CAD build for the part. Positions are in the model's coordinates, mm. A direction names the side the tool comes from. Give positions to 0.01 mm unless a question says otherwise; leave off trailing zeros. Write each loop counter-clockwise with the first axis right and the second up, starting at its lowest first coordinate (ties: lowest second). Pieces come first, ordered by that corner, then holes. Notation, with made-up numbers: (38, -15.5) - (76, -15.5) arc R8 cw to (76, -8.5) - close; hole circle Ø4 at (10.25, -20.75). An arc over 180 degrees is marked (long way). Answer as a JSON object with one key per item and string values.
from build123d import *

# Parameters (mm, degrees)
F0_W     = 461.772
F0_H     = 76.2
F1_DEPTH = 35.814
F2_W     = 62.3316
F2_H     = 31.496
F3_DEPTH = 461.773


with BuildPart() as f1:
    # F0 (on Top) → F1 (new body)
    with BuildSketch(Plane.XY):
        with Locations((-38.690397, 9.206371)):
            Rectangle(F0_W, F0_H)
    extrude(amount=F1_DEPTH)

    # F2 (on face) → F3 (cut, through all)
    with BuildSketch(Plane(origin=(-269.576397, 0, 0), x_dir=(0, -1, 0), z_dir=(-1, 0, 0))):
        with Locations((-9.206371, 20.066)):
            Rectangle(F2_W, F2_H)
    extrude(amount=-F3_DEPTH, mode=Mode.SUBTRACT)


solid = f1.part
(1) Saw through at B-B, the plane x = 6.5. Give the cut face in (y, z).
Answer key:
{"outline": "(-28.89, 0) - (47.31, 0) - (47.31, 35.81) - (40.37, 35.81) - (40.37, 4.32) - (-21.96, 4.32) - (-21.96, 35.81) - (-28.89, 35.81) - close"}
(2) Pull direction Y, two halves, no side cores. Call faces 1 (the face through (-269.576, 3, 3)), 2 (the face through (-42, 47.306, 18)), 3 (the face through (-42, -21.959, 20)): pulls with the +Y half, pulls with the -Y half, needs draft (parallel to the pull), parting line crosses it, or undercut.
Answer key:
{"face 1": "needs draft", "face 2": "pulls with the +Y half", "face 3": "undercut"}
(3) Flat gauge pin, fed straight in: P1, Ø5, axis at y = 37, z = 7.5, coming from the -X side. Where does the tip first touch, or does it go through?
Answer key:
{"P1": "passes through"}
(4) Probe L1, parallel to Y at x = 117, z = 17; L2, parallel to Z at x = -116.5, y = 35.5. List the from-to ranges inside material, lowest first. Write a range as [from, to].
Answer key:
{"L1": "y = [-28.89, -21.96], [40.37, 47.31]", "L2": "z = [0, 4.32]"}
(5) Saw through at C-C, the plane y = -1. Give the cut face in (x, z), and give its area (3 significant figures).
Answer key:
{"outline": "(-269.58, 0) - (192.2, 0) - (192.2, 4.32) - (-269.58, 4.32) - close", "area": "1,990 mm²"}
(6) Saw through at A-A, the plane z = 20.5. Give the cut face in (x, y), and give its area (3 significant figures).
Answer key:
{"outline": "(-269.58, -28.89) - (192.2, -28.89) - (192.2, -21.96) - (-269.58, -21.96) - close; (-269.58, 40.37) - (192.2, 40.37) - (192.2, 47.31) - (-269.58, 47.31) - close", "area": "6,400 mm²"}
(7) 3-axis set-ups, long thin cutter, end or side, ignore diameter. For faces 4 (the face through (-42, -28.894, 18)), 5 (the face through (-42, 10, 4.318)): which of +Z, -Z, +X, -X, +Y, -Y reach the whole face in a straight line?
Answer key:
{"face 4": "+Z, -Z, +X, -X, -Y", "face 5": "+Z, +X, -X"}
